Here's how the part is built. I have some questions about the finished solid (model axes, mm). Face numbers are marked on the shaded views. A direction names the side the tool comes from. Round coordinates to 2 decimals unless told otherwise and drop trailing zeros. Write each loop counter-clockwise with the first axis right and the second up, starting at its lowest first coordinate (ties: lowest second). Pieces come first, ordered by that corner, then holes. Notation, with made-up numbers: (71, -13) -> (116, -13) arc R22 cw to (116, 7) -> close; hole circle Ø4 at (11.25, -13.75). An arc over 180 degrees is marked (long way). Put each result on its own line as item: value. Start each with the question number.
1. Suppose I cut it at B-B (x = -41.5). Please give me the cut outline in (y, z).
2. Which directions (+Z, -Z, +X, -X, +Y, -Y) give clear straight access to the entire face, cutting with the end or side of a thin tool? Please do the marked faces 3, 4, 5 and 6.
3. For pin 1 (10 mm diameter, centred on x = 7, y = -10.5, fed in from +Z); pin 2 (6 mm diameter, centred on x = -13, z = -23.5, fed in from +Y); pin 3 (1 mm diameter, centred on x = -10.5, y = 9, fed in from -Z), each with a flat end and sliding along its axis, tell me the tip position at first contact or that it passes through.
4. We'd pull the mould along Z, two halves only. Please class the marked faces 1 and 2: +Z half, -Z half, draft (parallel to the pull), parting line (faces both ways), or undercut.
5. I need wall thicknesses on probe 1 along Z at (x, y) = (0, 18.5); probe 2 along X at (y, z) = (37.5, -11.5). Which ranges of each line are inside material? Lowest first, please. Write a range as from..to.
6. Suppose I cut it at A-A (z = -18). Count the separate pieces of the cut face and the enclosed holes in it, then the cut area to 3 significant figures.
```python
from build123d import *

# Parameters (mm, degrees)
SKETCH5_R           = 30.3149
BOSS_EXTRUDE1_DEPTH = 68.1228
SKETCH6_R           = 30.3149
BOSS_EXTRUDE2_DEPTH = 34.0614
FILLET1_R           = 3.048


with BuildPart() as part:
    # Sketch1 → Revolve1 (revolve)
    with BuildSketch(Plane.XY):
        Polygon((-38.1, -34.3535), (-34.0614, -30.3149), (-34.0614, -26.2509), (-38.1, -30.099), (-57.15, -30.2895), (-57.15, -34.3535), align=None)
    revolve(axis=Axis((-57.15, 0, 0), (1, 0, 0)))


with BuildPart() as body_2:
    # Mirror1: mirrored copy
    add(part.part.mirror(Plane(origin=(0, 0, 0), x_dir=(0, 0, 1), z_dir=(1, 0, 0))))


with BuildPart() as body_3:
    # Sketch2 → Revolve2 (revolve)
    with BuildSketch(Plane.XY):
        Polygon((30.2895, 57.15), (30.099, 38.1), (26.2509, 34.0614), (30.3149, 34.0614), (34.3535, 38.1), (34.3535, 57.15), align=None)
    revolve(axis=Axis((0, 0, 0), (0, 1, 0)))


with BuildPart() as part_1:
    add(part.part)

    add(body_2.part)  # Boss-Extrude1 merges body 2
    # Sketch5 → Boss-Extrude1 (add)
    with BuildSketch(Plane(origin=(-34.0614, 0, 0), x_dir=(0, 0, -1), z_dir=(1, 0, 0))):
        Circle(SKETCH5_R)
    extrude(amount=BOSS_EXTRUDE1_DEPTH)

    add(body_3.part)  # Boss-Extrude2 merges body 3
    # Sketch6 → Boss-Extrude2 (add)
    with BuildSketch(Plane.XZ.offset(-34.0614)):
        Circle(SKETCH6_R)
    extrude(amount=BOSS_EXTRUDE2_DEPTH)

    # Fillet1
    fillet1_edges = [part_1.edges().sort_by_distance(p)[0] for p in [
        (-34.0614, 21.435871361, 21.435871361),
        (34.0614, 21.435871361, 21.435871361),
        (-38.1, 34.3535, 0),
        (38.1, 34.3535, 0),
        (-30.3149, 34.0614, 0),
        (-34.3535, 38.1, 0),
    ]]
    fillet(fillet1_edges, radius=FILLET1_R)

    # Sketch7 → Cut-Revolve1 (revolve, cut)
    with BuildSketch(Plane.XY):
        Polygon((-57.15, 0), (57.15, 0), (57.15, 30.2895), (38.1, 30.099), (34.0614, 26.2509), (-34.0614, 26.2509), (-38.1, 30.099), (-57.15, 30.2895), align=None)
    revolve(axis=Axis((-57.15, 0, 0), (1, 0, 0)), mode=Mode.SUBTRACT)

    # Sketch8 → Cut-Revolve4 (revolve, cut)
    with BuildSketch(Plane.XY):
        Polygon((30.2895, 57.15), (30.099, 38.1), (26.2509, 34.0614), (26.2509, 0), (0, 0), (0, 57.15), align=None)
    revolve(axis=Axis((0, 0, 0), (0, 1, 0)), mode=Mode.SUBTRACT)


solid = part_1.part
```
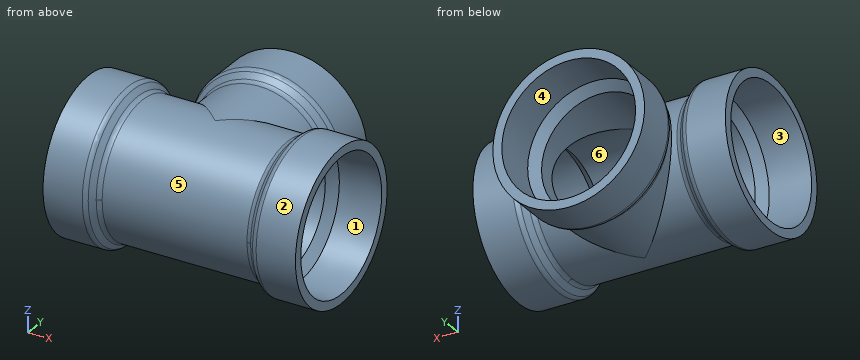
Verdict:
1. outline: circle Ø68.71 at (0, 0); hole circle Ø60.27 at (0, 0)
2. face 3: -X
2. face 4: +Y
2. face 5: none
2. face 6: +X, -X
3. pin 1: stops at z = 29.81
3. pin 2: stops at y = 37.85
3. pin 3: stops at z = -29.1
4. face 1: undercut
4. face 2: parting line
5. probe 1: z = -30.31..-26.25, 26.25..30.31
5. probe 2: x = -31.7..-27.2, 27.2..31.7
6. separate pieces: 3
6. enclosed holes: 0
6. area: 1,320 mm^2
